```python
from build123d import *

# Parameters (mm, degrees)
BOSS_EXTRUDE1_DEPTH = 3
FILLET4_R           = 7
FILLET5_R           = 7
FILLET6_R           = 7
SKETCH6_R           = 10
BOSS_EXTRUDE2_DEPTH = 1
SKETCH10_W          = 3
SKETCH10_H          = 15
BOSS_EXTRUDE3_DEPTH = 9
SKETCH11_R          = 1.5
CUT_EXTRUDE4_DEPTH  = 14
SKETCH13_R          = 1.5
CUT_EXTRUDE5_DEPTH  = 10


with BuildPart() as part:
    # Sketch1 → Boss-Extrude1 (new body)
    with BuildSketch(Plane.XY):
        Polygon((0, 0), (80, 0), (40, 69.282032303), align=None)
    extrude(amount=BOSS_EXTRUDE1_DEPTH)

    # Fillet4
    fillet4_edges = [part.edges().sort_by_distance(p)[0] for p in [
        (0, 0, 1.5),
    ]]
    fillet(fillet4_edges, radius=FILLET4_R)

    # Fillet5
    fillet5_edges = [part.edges().sort_by_distance(p)[0] for p in [
        (80, 0, 1.5),
    ]]
    fillet(fillet5_edges, radius=FILLET5_R)

    # Fillet6
    fillet6_edges = [part.edges().sort_by_distance(p)[0] for p in [
        (40, 69.282032303, 1.5),
    ]]
    fillet(fillet6_edges, radius=FILLET6_R)

    # Sketch6 → Boss-Extrude2 (add)
    with BuildSketch(Plane(origin=(0, 0, 0), x_dir=(-1, 0, 0), z_dir=(0, 0, -1))):
        with Locations(Location((-40, 44.282032303, 0), (0, 0, 180))):
            Circle(SKETCH6_R)
        with Locations(Location((-58.349364905, 12.5, 0), (0, 0, 180))):
            Circle(SKETCH6_R)
        with Locations(Location((-21.650635095, 12.5, 0), (0, 0, 180))):
            Circle(SKETCH6_R)
    extrude(amount=BOSS_EXTRUDE2_DEPTH)

    # Sketch7 → Cut-Revolve2 (revolve, cut)
    with BuildSketch(Plane(origin=(0, 0, -1.5), x_dir=(-1, 0, 0), z_dir=(0, 0, -1))):
        with BuildLine():
            Line((-40, 52.282032303), (-40, 36.282032303))
            ThreePointArc((-40, 36.282032303), (-32, 44.282032303), (-40, 52.282032303))
        make_face()
    revolve(axis=Axis((40, 52.282032303, -1.5), (0, -1, 0)), mode=Mode.SUBTRACT)

    # Sketch8 → Cut-Revolve3 (revolve, cut)
    with BuildSketch(Plane(origin=(0, 0, -1), x_dir=(-1, 0, 0), z_dir=(0, 0, -1))):
        with BuildLine():
            Line((-58.349364905, 20.5), (-58.349364905, 4.5))
            ThreePointArc((-58.349364905, 4.5), (-50.349364905, 12.5), (-58.349364905, 20.5))
        make_face()
    revolve(axis=Axis((58.349364905, 20.5, -1), (0, -1, 0)), mode=Mode.SUBTRACT)

    # Sketch9 → Cut-Revolve4 (revolve, cut)
    with BuildSketch(Plane(origin=(0, 0, -1), x_dir=(-1, 0, 0), z_dir=(0, 0, -1))):
        with BuildLine():
            Line((-21.650635095, 20.5), (-21.650635095, 4.5))
            ThreePointArc((-21.650635095, 4.5), (-13.650635095, 12.5), (-21.650635095, 20.5))
        make_face()
    revolve(axis=Axis((21.650635095, 20.5, -1), (0, -1, 0)), mode=Mode.SUBTRACT)

    # Sketch10 → Boss-Extrude3 (add)
    with BuildSketch(Plane(origin=(0, 0, 0), x_dir=(-1, 0, 0), z_dir=(0, 0, -1))):
        with Locations((-35.5, 21.828790282)):
            Rectangle(SKETCH10_W, SKETCH10_H)
        with Locations((-44.5, 21.828790282)):
            Rectangle(SKETCH10_W, SKETCH10_H)
    extrude(amount=BOSS_EXTRUDE3_DEPTH)

    # Sketch11 → Cut-Extrude4 (cut)
    with BuildSketch(Plane.ZY.offset(-34)):
        with Locations((-4.5, 24.828790282)):
            Circle(SKETCH11_R)
        with Locations((-4.5, 18.828790282)):
            Circle(SKETCH11_R)
    extrude(amount=-CUT_EXTRUDE4_DEPTH, mode=Mode.SUBTRACT)

    # Sketch13 → Cut-Extrude5 (cut)
    with BuildSketch(Plane.XY.offset(3)):
        with Locations((40, 21.828790282)):
            Circle(SKETCH13_R)
    extrude(amount=-CUT_EXTRUDE5_DEPTH, mode=Mode.SUBTRACT)


solid = part.part
```
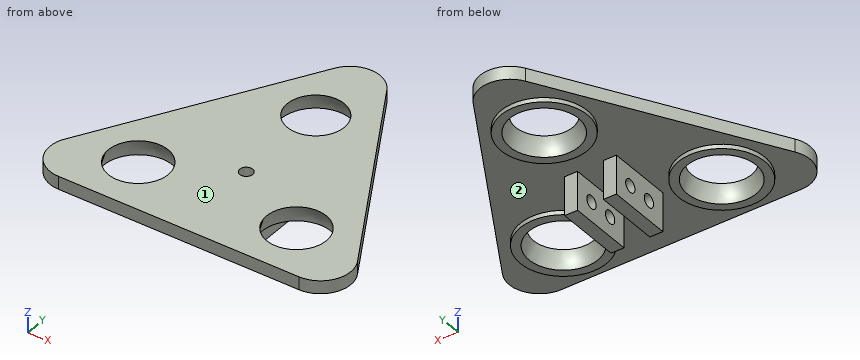
Could you check a few things on this model? Use its own coordinates, in mm. Face numbers are marked on the shaded views. Give positions to 0.01 mm unless a question says otherwise; leave off trailing zeros. Write each loop counter-clockwise with the first axis right and the second up, starting at its lowest first coordinate (ties: lowest second). Pieces come first, ordered by that corner, then holes. Notation, with made-up numbers: (65.25, -13) - (115.25, -13) arc R21 cw to (115.25, 13) - close; hole circle Ø6 at (1, 21). An arc over 180 degrees is marked (long way). One line per item, written item: value. Start each with the question number.
Item 1: Imagine slicing it at D-D, the plane y = 47.5. List the corners of the cut face in (x, z) for me.
Item 2: I'm going to push flat-ended pins straight in: pin 1 (3.5 mm diameter, centred on x = 36, z = -5, fed in from -Y); pin 2 (3 mm diameter, centred on x = 35, y = 55.5, fed in from -Z); pin 3 (2 mm diameter, centred on y = 22.5, z = 1, fed in from +X). Where does each tip first touch, or does it pass through?
Item 3: If we mould it in two halves opening along X, with no side actions, what happens to the marked faces 1 and 2? For each: +X half, -X half, draft (parallel to the pull), parting line (faces both ways), or undercut.
Item 4: Imagine slicing it at A-A, the plane y = 12.5. List the corners of the cut face in (x, z) for me.
Item 5: Imagine slicing it at C-C, the plane x = 20.5. List the corners of the cut face in (y, z) for me, and give its area (3 significant figures).
Item 6: Please list where these lines run through material, in increasing order: line 1 (Y direction, x = 45.35, z = -4.5); line 2 (Y direction, x = 40, z = 1); line 3 (Z direction, x = 23, y = 26). Write a range as from..to.
Item 7: Imagine slicing it at B-B, the plane z = -4.5. List the corners of the cut face in (x, y) for me.
Geometry says:
1. outline: (27.42, 0) - (30.53, 0) - (30.53, -1) - (32.69, -1) arc R7.32 cw to (34.22, 3) - (27.42, 3) - close; (45.78, 3) arc R7.32 cw to (47.31, -1) - (49.47, -1) - (49.47, 0) - (52.58, 0) - (52.58, 3) - close
2. pin 1: y = 14.33
2. pin 2: z = 0
2. pin 3: x = 67.59
3. face 1: draft
3. face 2: undercut
4. outline: (7.22, 0) - (11.65, 0) - (11.65, -1) - (13.65, -1) arc R8 cw to (14.72, 3) - (7.22, 3) - close; (28.58, 3) arc R8 cw to (29.65, -1) - (31.65, -1) - (31.65, 0) - (48.35, 0) - (48.35, -1) - (50.35, -1) arc R8 cw to (51.42, 3) - close; (65.28, 3) arc R8 cw to (66.35, -1) - (68.35, -1) - (68.35, 0) - (72.78, 0) - (72.78, 3) - close
5. outline: (0, 0) - (2.57, 0) - (2.57, -1) - (4.58, -1) arc R7.92 cw to (5.67, 3) - (0, 3) - close; (19.33, 3) arc R7.92 cw to (20.42, -1) - (22.43, -1) - (22.43, 0) - (35.51, 0) - (35.51, 3) - close
5. area: 65.9 mm^2
6. line 1: 14.33..17.33, 20.33..23.33, 26.33..29.33
6. line 2: 0..20.33, 23.33..36.68, 51.88..62.28
6. line 3: 0..3
7. outline: (34, 14.33) - (37, 14.33) - (37, 17.33) - (34, 17.33) - close; (34, 20.33) - (37, 20.33) - (37, 23.33) - (34, 23.33) - close; (34, 26.33) - (37, 26.33) - (37, 29.33) - (34, 29.33) - close; (43, 14.33) - (46, 14.33) - (46, 17.33) - (43, 17.33) - close; (43, 20.33) - (46, 20.33) - (46, 23.33) - (43, 23.33) - close; (43, 26.33) - (46, 26.33) - (46, 29.33) - (43, 29.33) - close
